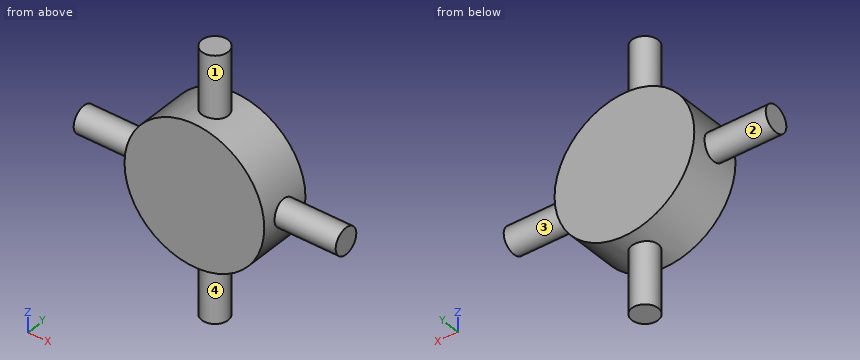
```python
from build123d import *

# Parameters (mm, degrees)
F0_R     = 10.16
F1_DEPTH = 3.81
F2_R     = 1.905
F3_DEPTH = 19.05
F4_R     = 1.905
F5_DEPTH = 19.05


with BuildPart() as f1:
    # F0 (on Front) → F1 (new body, symmetric)
    with BuildSketch(Plane.XZ):
        Circle(F0_R)
    extrude(amount=F1_DEPTH, both=True)

    # F2 (on Top) → F3 (join, symmetric)
    with BuildSketch(Plane.XY):
        Circle(F2_R)
    extrude(amount=F3_DEPTH, both=True)

    # F4 (on Right) → F5 (join, symmetric)
    with BuildSketch(Plane.YZ):
        Circle(F4_R)
    extrude(amount=F5_DEPTH, both=True)


solid = f1.part
```
The listing builds one solid part. Answer for the finished solid, in the listing's coordinates (mm). Face numbers are marked on the shaded views. A direction names the side the tool comes from. Coordinates: 2 decimals unless noted, no trailing zeros. Loops run counter-clockwise (first coordinate to the right, second up) from the corner with the lowest first, then second, coordinate; pieces in that order, holes last. Notation, with made-up numbers: M 79,-25.75 L 138,-25.75 A30 cw 138,10.25 Z; hole C -36.75,23 d10. An arc over 180 degrees is marked long. Answer as CSV lines item,"result". Start each with the question number.
(1) The part is cut by section C-C (z = 0). Give the vertices of the cut face in (x, y) (3 decimals), and give its area (3 significant figures).
(2) The part is cut by section B-B (x = 0). Give the vertices of the cut face in (y, z) (3 decimals).
(3) Given pin 1 (4 mm diameter, centred on y = -2, z = -0.5, fed in from +X), flat-ended and moving along its own axis, determine where the tip first touches the part or whether it passes through.
(4) Find the intervals of material crossed by L1, parallel to X at y = 2, z = 0; L2, parallel to X at y = 0, z = 16.5 (3 decimals); L3, parallel to Z at x = 11.5, y = 0.75, in increasing order. Write a range as [from, to].
(5) The part is cut by section A-A (y = 0). Give the vertices of the cut face in (x, z) (3 decimals).
(6) The part is cut by section D-D (y = -2.75). Give the vertices of the cut face in (x, z), and give its area (3 significant figures).
(7) For the marked faces 1, 2, 3 and 4, determine the directions among +Z, -Z, +X, -X, +Y, -Y from which every point of the face is accessible in a straight line to the end or side of a thin tool.
Determined:
1,outline,"M -19.05,-1.905 L -10.16,-1.905 L -10.16,-3.81 L 10.16,-3.81 L 10.16,-1.905 L 19.05,-1.905 L 19.05,1.905 L 10.16,1.905 L 10.16,3.81 L -10.16,3.81 L -10.16,1.905 L -19.05,1.905 Z"
1,area,"223 mm2"
2,outline,"M -3.81,-10.16 L -1.905,-10.16 L -1.905,-19.05 L 1.905,-19.05 L 1.905,-10.16 L 3.81,-10.16 L 3.81,10.16 L 1.905,10.16 L 1.905,19.05 L -1.905,19.05 L -1.905,10.16 L -3.81,10.16 Z"
3,pin 1,"x = 19.05"
4,L1,"[-10.16, 10.16]"
4,L2,"[-1.905, 1.905]"
4,L3,"[-1.75, 1.75]"
5,outline,"M -19.05,-1.905 L -9.98,-1.905 A10.16 ccw -1.905,-9.98 L -1.905,-19.05 L 1.905,-19.05 L 1.905,-9.98 A10.16 ccw 9.98,-1.905 L 19.05,-1.905 L 19.05,1.905 L 9.98,1.905 A10.16 ccw 1.905,9.98 L 1.905,19.05 L -1.905,19.05 L -1.905,9.98 A10.16 ccw -9.98,1.905 L -19.05,1.905 Z"
6,outline,"C 0,0 d20.32"
6,area,"324 mm2"
7,face 1,"+Z"
7,face 2,"-X"
7,face 3,"+X"
7,face 4,"-Z"
